```python
from build123d import *

# Parameters (mm, degrees)
SKETCH2_W           = 24
SKETCH2_H           = 14
BOSS_EXTRUDE1_DEPTH = 4.5
SKETCH3_W           = 14
SKETCH3_H           = 14
BOSS_EXTRUDE2_DEPTH = 5
CUT_EXTRUDE1_DEPTH  = 10
SKETCH5_W           = 10
SKETCH5_H           = 7.54749529
CUT_EXTRUDE2_DEPTH  = 7.5
SKETCH6_W           = 12.5
SKETCH6_H           = 1.6
CUT_EXTRUDE3_DEPTH  = 4
SKETCH7_W           = 10.060724294
SKETCH7_H           = 1.6
CUT_EXTRUDE4_DEPTH  = 1
SKETCH8_W           = 0.45250471
SKETCH8_H           = 1.6
CUT_EXTRUDE5_DEPTH  = 0.025884761
SKETCH9_W           = 1
SKETCH9_H           = 1.6
BOSS_EXTRUDE3_DEPTH = 0.086609054
FILLET1_R           = 1
FILLET2_R           = 1
FILLET3_R           = 1


with BuildPart() as part:
    # Sketch2 → Boss-Extrude1 (new body)
    with BuildSketch(Plane(origin=(0, 0, 0), x_dir=(1, 0, 0), z_dir=(0, 1, 0))):
        with Locations((2.394366197, 1.248826291)):
            Rectangle(SKETCH2_W, SKETCH2_H)
    extrude(amount=BOSS_EXTRUDE1_DEPTH)

    # Sketch3 → Boss-Extrude2 (add)
    with BuildSketch(Plane(origin=(0, 4.5, 0), x_dir=(1, 0, 0), z_dir=(0, 1, 0))):
        with Locations((2.394366197, 1.248826291)):
            Rectangle(SKETCH3_W, SKETCH3_H)
    extrude(amount=BOSS_EXTRUDE2_DEPTH)

    # Sketch4 → Cut-Extrude1 (cut)
    with BuildSketch(Plane(origin=(0, 0, -8.248826291), x_dir=(-1, 0, 0), z_dir=(0, 0, -1))):
        Polygon((-4.994366197, 4.2), (-4.994366197, 2), (0.205633803, 2), (0.205633803, 4.2), (0.205633803, 10.153994243), (-4.994366197, 10.153994243), align=None)
    extrude(amount=-CUT_EXTRUDE1_DEPTH, mode=Mode.SUBTRACT)

    # Sketch5 → Cut-Extrude2 (cut)
    with BuildSketch(Plane(origin=(0, 9.5, 0), x_dir=(1, 0, 0), z_dir=(0, 1, 0))):
        with Locations((2.394366197, 0.022573936)):
            Rectangle(SKETCH5_W, SKETCH5_H)
    extrude(amount=-CUT_EXTRUDE2_DEPTH, mode=Mode.SUBTRACT)

    # Sketch6 → Cut-Extrude3 (cut)
    with BuildSketch(Plane(origin=(0, 0, -8.248826291), x_dir=(-1, 0, 0), z_dir=(0, 0, -1))):
        with Locations((-2.394366197, 8.7)):
            Rectangle(SKETCH6_W, SKETCH6_H)
    extrude(amount=-CUT_EXTRUDE3_DEPTH, mode=Mode.SUBTRACT)

    # Sketch7 → Cut-Extrude4 (cut)
    with BuildSketch(Plane(origin=(0, 0, -4.248826291), x_dir=(-1, 0, 0), z_dir=(0, 0, -1))):
        with Locations((-2.33811929, 8.7)):
            Rectangle(SKETCH7_W, SKETCH7_H)
    extrude(amount=-CUT_EXTRUDE4_DEPTH, mode=Mode.SUBTRACT)

    # Sketch8 → Cut-Extrude5 (cut)
    with BuildSketch(Plane.ZY.offset(-7.368481437)):
        with Locations((-4.022573936, 8.7)):
            Rectangle(SKETCH8_W, SKETCH8_H)
    extrude(amount=-CUT_EXTRUDE5_DEPTH, mode=Mode.SUBTRACT)

    # Sketch9 → Boss-Extrude3 (add)
    with BuildSketch(Plane(origin=(-2.692242857, 0, 0), x_dir=(0, 0, -1), z_dir=(1, 0, 0))):
        with Locations((3.748826291, 8.7)):
            Rectangle(SKETCH9_W, SKETCH9_H)
    extrude(amount=BOSS_EXTRUDE3_DEPTH)

    # Fillet1
    fillet1_edges = [part.edges().sort_by_distance(p)[0] for p in [
        (14.394366197, 4.5, -1.248826291),
        (2.394366197, 9.5, 5.751173709),
        (-9.605633803, 4.5, -1.248826291),
        (14.394366197, 0, -1.248826291),
        (-9.605633803, 0, -1.248826291),
    ]]
    fillet(fillet1_edges, radius=FILLET1_R)

    # Fillet2
    fillet2_edges = [part.edges().sort_by_distance(p)[0] for p in [
        (-6.605633803, 4.5, -8.248826291),
        (-9.605633803, 2.25, -8.248826291),
        (2.394366197, 0, -8.248826291),
        (11.394366197, 4.5, -8.248826291),
        (14.394366197, 2.25, -8.248826291),
        (14.101472978, 4.207106781, -8.248826291),
        (14.101472978, 0.292893219, -8.248826291),
        (-9.312740584, 4.207106781, -8.248826291),
        (-9.312740584, 0.292893219, -8.248826291),
    ]]
    fillet(fillet2_edges, radius=FILLET2_R)

    # Fillet3
    fillet3_edges = [part.edges().sort_by_distance(p)[0] for p in [
        (-0.205633803, 4.95, -3.796321581),
        (4.994366197, 4.95, -3.796321581),
    ]]
    fillet(fillet3_edges, radius=FILLET3_R)


solid = part.part
```
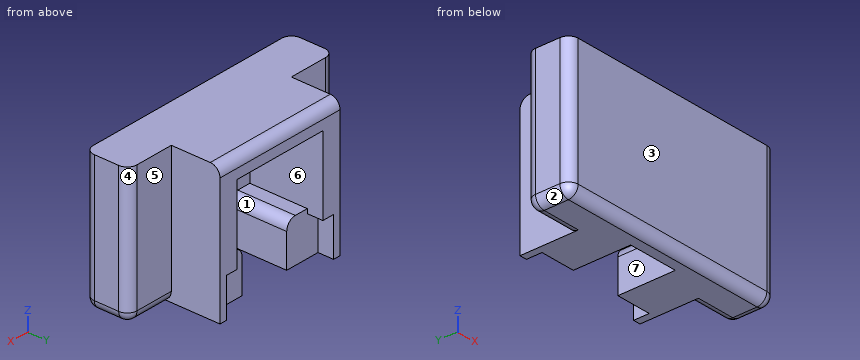
Model file for the job. Use its own axes, mm. Face numbers are marked on the shaded views. A direction names the side the tool comes from. Coordinates: 2 decimals unless noted, no trailing zeros. Loops run counter-clockwise (first coordinate to the right, second up) from the corner with the lowest first, then second, coordinate; pieces in that order, holes last. Notation, with made-up numbers: (24.25, 59.25) - (29.25, 59.25) arc R27 ccw to (29.25, 88.25) - close; hole circle Ø11 at (44.5, 88.5). An arc over 180 degrees is marked (long way). Answer as a JSON object with one key per item and string values. Group by question number.
(1) Cut at C-C (y = 3.25). Give the cut face in (x, z), then the cut area to 3 significant figures.
(2) Tool access for the marked faces 5, 6 and 7: list every direction of +Z, -Z, +X, -X, +Y, -Y with a clear straight run to the whole face (end or side of a thin tool).
(3) Cut at D-D (z = -0.25). Give the cut face in (x, y), then the cut area to 3 significant figures.
(4) Flat gauge pins, fed straight in: pin 1 (8 mm diameter, centred on x = 1.5, z = -2, fed in from +Y); pin 2 (1 mm diameter, centred on y = 4.5, z = -7, fed in from +X); pin 3 (3 mm diameter, centred on y = 8.5, z = -6.5, fed in from -X). Where does each tip first touch, or does it go through?
(5) Cut at A-A (x = 2.25). Give the cut face in (y, z), then the cut area to 3 significant figures.
(6) Cut at B-B (z = -6.5). Give the cut face in (x, y).
(7) Probe line 1 along X through (y, z) = (6, 2); line 2 along X through (y, z) = (2.75, -4.75); line 3 along Y through (x, z) = (-3, -6.5). List the from-to ranges inside material, lowest first.
(8) Two-plate mould, pull along X, no slides. Class the marked faces 1, 2, 3 and 4: released by +X, released by -X, zero draft, split by the parting line, or undercut.
Geometry says:
{
 "1": {"outline": "(-9.61, -7.25) arc R1 ccw to (-8.61, -8.25) - (-0.21, -8.25) - (-0.21, -4.8) arc R1 ccw to (-1.21, -3.8) - (-2.61, -3.8) - (-2.61, 3.75) - (7.39, 3.75) - (7.39, -3.8) - (5.99, -3.8) arc R1 ccw to (4.99, -4.8) - (4.99, -8.25) - (13.39, -8.25) arc R1 ccw to (14.39, -7.25) - (14.39, 5.75) - (-9.61, 5.75) - close", "area": "237 mm^2"},
 "2": {"face 5": "+Z, -Z, +X, +Y", "face 6": "+Y", "face 7": "-Z, +Y"},
 "3": {"outline": "(-9.61, 1) arc R1 ccw to (-8.61, 0) - (13.39, 0) arc R1 ccw to (14.39, 1) - (14.39, 3.5) arc R1 ccw to (13.39, 4.5) - (9.39, 4.5) - (9.39, 9.5) - (7.39, 9.5) - (7.39, 2) - (-2.61, 2) - (-2.61, 9.5) - (-4.61, 9.5) - (-4.61, 4.5) - (-8.61, 4.5) arc R1 ccw to (-9.61, 3.5) - close", "area": "102 mm^2"},
 "4": {"pin 1": "stops at y = 7.9", "pin 2": "stops at x = 14.26", "pin 3": "stops at x = -4.61"},
 "5": {"outline": "(0, -7.25) arc R1 ccw to (1, -8.25) - (2, -8.25) - (2, 3.75) - (9.5, 3.75) - (9.5, 4.75) arc R1 ccw to (8.5, 5.75) - (0, 5.75) - close", "area": "42.6 mm^2"},
 "6": {"outline": "(-9.61, 1) arc R1 ccw to (-8.61, 0) - (13.39, 0) arc R1 ccw to (14.39, 1) - (14.39, 3.5) arc R1 ccw to (13.39, 4.5) - (9.39, 4.5) - (9.39, 9.5) - (8.64, 9.5) - (8.64, 7.9) - (4.99, 7.9) - (4.99, 2) - (-0.21, 2) - (-0.21, 7.9) - (-3.86, 7.9) - (-3.86, 9.5) - (-4.61, 9.5) - (-4.61, 4.5) - (-8.61, 4.5) arc R1 ccw to (-9.61, 3.5) - close"},
 "7": {"line 1": "x = -4.61 to -2.61, 7.39 to 9.39", "line 2": "x = -9.61 to -0.21, 5 to 14.39", "line 3": "y = 0 to 7.9"},
 "8": {"face 1": "undercut", "face 2": "released by -X", "face 3": "zero draft", "face 4": "released by +X"}
}
